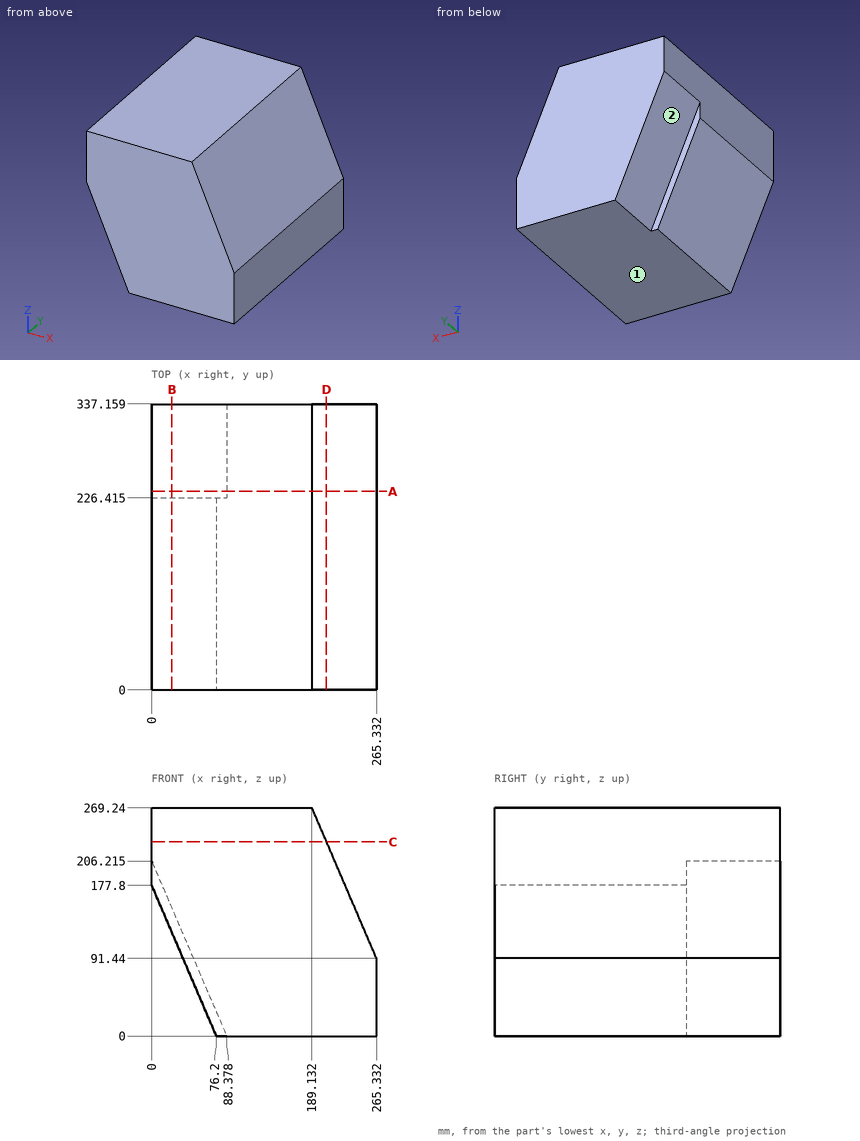
Part print with two shaded views. Sizes in mm from the minimum x, y, z corner. A direction names the side the tool comes from. Coordinates: 2 decimals unless noted, no trailing zeros. Order: outer loops, then holes, each group sorted by start corner. A loop starts at its lowest first (then second) coordinate and runs counter-clockwise, first axis right, second up. Notation, with made-up numbers: (-2.5, 5.5) - (54.5, 5.5) arc R19 cw to (54.5, 9.5) - close; hole circle Ø3 at (-29, 30). An arc over 180 degrees is marked (long way). Answer in a Markdown table with one row per item.
1. 3-axis set-ups, long thin cutter, end or side, ignore diameter. For the marked faces 1 and 2: which of +Z, -Z, +X, -X, +Y, -Y reach the whole face in a straight line?
Answer:
| item | result |
|---|---|
| face 1 | -Z, +X, -X, +Y, -Y |
| face 2 | -Z, -X, +Y |
2. Slice it at B-B, the plane x = 24. List the corners of the cut face in (y, z) (1 decimal).
Answer:
| item | result |
|---|---|
| outline | (0, 121.8) - (226.4, 121.8) - (226.4, 150.2) - (337.2, 150.2) - (337.2, 269.2) - (0, 269.2) - close |
3. Slice it at C-C, the plane z = 229. List the corners of the cut face in (x, y), then the cut area to 3 significant figures.
Answer:
| item | result |
|---|---|
| outline | (0, 0) - (206.38, 0) - (206.38, 337.16) - (0, 337.16) - close |
| area | 69,600 mm² |
4. Flat gauge pin, fed straight in: P1, Ø4, axis at y = 242.5, z = 75.5, coming from the -X side. Where does the tip first touch, or does it go through?
Answer:
| item | result |
|---|---|
| P1 | x = 55.16 |
5. Drill centre lines: L1, parallel to X at y = 177.5, z = 222; L2, parallel to Z at x = 68.5, y = 132 (1 decimal); L3, parallel to Z at x = 70, y = 87 (1 decimal). Where is each one in solid material? Low to high. Write a range as from..to.
Answer:
| item | result |
|---|---|
| L1 | 0..209.38 |
| L2 | 18..269.2 |
| L3 | 14.5..269.2 |
6. Slice it at D-D, the plane x = 206. List the corners of the cut face in (y, z).
Answer:
| item | result |
|---|---|
| outline | (0, 0) - (337.16, 0) - (337.16, 229.88) - (0, 229.88) - close |
7. Slice it at A-A, the plane y = 234. List the corners of the cut face in (x, z) (1 decimal), then the cut area to 3 significant figures.
Answer:
| item | result |
|---|---|
| outline | (0, 206.2) - (88.4, 0) - (265.3, 0) - (265.3, 91.4) - (189.1, 269.2) - (0, 269.2) - close |
| area | 55,600 mm² |
